Geometry: final body of the model. Coordinates: model frame, mm. A direction names the side the tool comes from. Coordinates: 2 decimals unless noted, no trailing zeros. Write each loop counter-clockwise with the first axis right and the second up, starting at its lowest first coordinate (ties: lowest second). Pieces come first, ordered by that corner, then holes. Notation, with made-up numbers: (2, 13.5) -> (6, 13.5) arc R8 cw to (6, 17.5) -> close; hole circle Ø9 at (-12, 62.5). An arc over 180 degrees is marked (long way). One line per item, written item: value.
```python
from build123d import *

# Parameters (mm, degrees)
SKETCH1_W            = 133
SKETCH1_H            = 41
BOSS_EXTRUDE1_DEPTH  = 12
SKETCH2_W            = 95
SKETCH2_H            = 12
BOSS_EXTRUDE2_DEPTH  = 15
FILLET1_R            = 2
M2_CLEARANCE_HOLE1_D = 2.4
VENT1_DEPTH          = 12
FILLET2_R            = 1


# Read off the part's stored shape, not the designer's step: Vent1
with BuildPart() as part:
    # Sketch1 → Boss-Extrude1 (new body)
    with BuildSketch(Plane.XY):
        Rectangle(SKETCH1_W, SKETCH1_H)
    extrude(amount=BOSS_EXTRUDE1_DEPTH)

    # Sketch2 → Boss-Extrude2 (add)
    with BuildSketch(Plane(origin=(0, 20.5, 0), x_dir=(1, 0, 0), z_dir=(0, 1, 0))):
        with Locations((-2, -6)):
            Rectangle(SKETCH2_W, SKETCH2_H)
    extrude(amount=BOSS_EXTRUDE2_DEPTH)

    # Fillet1
    fillet1_edges = [part.edges().sort_by_distance(p)[0] for p in [
        (-49.5, 35.5, 6),
        (45.5, 35.5, 6),
        (-66.5, 20.5, 6),
        (66.5, 20.5, 6),
        (66.5, -20.5, 6),
        (-66.5, -20.5, 6),
    ]]
    fillet(fillet1_edges, radius=FILLET1_R)

    # M2 Clearance Hole1 (through all)
    with Locations(Plane(origin=(-42, 27, 12), x_dir=(1, 0, 0), z_dir=(0, 0, 1))):
        with Locations((0, 0), (80, 0)):
            Hole(M2_CLEARANCE_HOLE1_D / 2)

    # Vent1 outline → Vent1 (cut)
    with BuildSketch(Plane.XY):
        Polygon((-39.847390778, 12.5), (-46.320873948, 12.5), (-58.5, 0.320873948), (-58.5, -6.152609222), align=None)
        Polygon((-26.302839797, 12.5), (-32.776322967, 12.5), (-57.776322967, -12.5), (-51.302839797, -12.5), align=None)
        Polygon((-12.758288815, 12.5), (-19.231771985, 12.5), (-44.231771985, -12.5), (-37.758288815, -12.5), align=None)
        Polygon((0.786262167, 12.5), (-5.687221003, 12.5), (-30.687221003, -12.5), (-24.213737833, -12.5), align=None)
        Polygon((14.330813149, 12.5), (7.857329979, 12.5), (-17.142670021, -12.5), (-10.669186851, -12.5), align=None)
        Polygon((27.875364131, 12.5), (21.401880961, 12.5), (-3.598119039, -12.5), (2.875364131, -12.5), align=None)
        Polygon((-53.39194176, 12.5), (-58.5, 12.5), (-58.5, 7.39194176), align=None)
        Polygon((41.419915112, 12.5), (34.946431942, 12.5), (9.946431942, -12.5), (16.419915112, -12.5), align=None)
        Polygon((54.964466094, 12.5), (48.490982924, 12.5), (23.490982924, -12.5), (29.964466094, -12.5), align=None)
        Polygon((37.035533906, -12.5), (43.509017076, -12.5), (58.5, 2.490982924), (58.5, 8.964466094), align=None)
        Polygon((50.580084888, -12.5), (58.5, -12.5), (58.5, -4.580084888), align=None)
    extrude(amount=VENT1_DEPTH, mode=Mode.SUBTRACT)

    # Fillet2
    fillet2_edges = [part.edges().sort_by_distance(p)[0] for p in [
        (50.580084888, -12.5, 6),
        (43.509017076, -12.5, 6),
        (58.5, 2.490982924, 6),
        (58.5, -4.580084888, 6),
        (37.035533906, -12.5, 6),
        (29.964466094, -12.5, 6),
        (54.964466094, 12.5, 6),
        (58.5, 8.964466094, 6),
        (23.490982924, -12.5, 6),
        (16.419915112, -12.5, 6),
        (41.419915112, 12.5, 6),
        (48.490982924, 12.5, 6),
        (9.946431942, -12.5, 6),
        (2.875364131, -12.5, 6),
        (27.875364131, 12.5, 6),
        (34.946431942, 12.5, 6),
        (14.330813149, 12.5, 6),
        (21.401880961, 12.5, 6),
        (-3.598119039, -12.5, 6),
        (-10.669186851, -12.5, 6),
        (0.786262167, 12.5, 6),
        (7.857329979, 12.5, 6),
        (-17.142670021, -12.5, 6),
        (-24.213737833, -12.5, 6),
        (-12.758288815, 12.5, 6),
        (-5.687221003, 12.5, 6),
        (-30.687221003, -12.5, 6),
        (-37.758288815, -12.5, 6),
        (-26.302839797, 12.5, 6),
        (-19.231771985, 12.5, 6),
        (-44.231771985, -12.5, 6),
        (-51.302839797, -12.5, 6),
        (-39.847390778, 12.5, 6),
        (-32.776322967, 12.5, 6),
        (-57.776322967, -12.5, 6),
        (-58.5, -6.152609222, 6),
        (-53.39194176, 12.5, 6),
        (-46.320873948, 12.5, 6),
        (-58.5, 0.320873948, 6),
        (-58.5, 7.39194176, 6),
        (58.5, -12.5, 6),
    ]]
    fillet(fillet2_edges, radius=FILLET2_R)


solid = part.part
```
(1) Pull-direction query (X, two-part tool) for faces 1 (the flat face through (-49.5, 27, 6)), 2 (the flat face through (51, 12.5, 6)), 3 (the flat face through (9.8, 0.9, 5.9)), 4 (the flat face through (-1, 8, 12)); classes: released by +X, released by -X, zero draft, split by the parting line, or undercut.
Responses:
face 1: released by -X
face 2: undercut
face 3: undercut
face 4: zero draft
(2) Section B-B (z = 1.5). State how many separate pieces and enclosed holes the cut face has, then the cut area to 3 significant figures.
Responses:
separate pieces: 1
enclosed holes: 13
area: 5,500 mm2
(3) Reachability of faces 5 (the flat face through (-44.408, 0.868, 5.916)), 6 (the flat face through (55, 20.5, 6)), 7 (the flat face through (-66.5, 0, 6)) from +Z, -Z, +X, -X, +Y, -Y: full face, straight path, thin tool, end or side. Return the list, or none.
Responses:
face 5: +Z, -Z
face 6: +Z, -Z, +X, +Y
face 7: +Z, -Z, -X, +Y, -Y
(4) Section A-A (y = 27). Return the cut outline in (x, z).
Responses:
outline: (-49.5, 0) -> (-43.2, 0) -> (-43.2, 12) -> (-49.5, 12) -> close; (-40.8, 0) -> (36.8, 0) -> (36.8, 12) -> (-40.8, 12) -> close; (39.2, 0) -> (45.5, 0) -> (45.5, 12) -> (39.2, 12) -> close
(5) Line query: line 1 (Y direction, x = -22, z = 4.5); line 2 (Y direction, x = 31, z = 7); line 3 (Y direction, x = -42, z = 9.5). Output: solid intervals per line, ascending. Write a range as [from, to].
Responses:
line 1: y = [-20.5, -10.29], [-3.81, 3.26], [9.73, 35.5]
line 2: y = [-20.5, -11.46], [-4.99, 2.08], [8.55, 35.5]
line 3: y = [-20.5, -12.48], [-10.27, -3.2], [3.28, 10.35], [12.47, 25.8], [28.2, 35.5]
(6) First-contact query: pin 1 (3 mm diameter, centred on x = -53.5, z = 3.5, fed in from +Y). Flat tip, straight axial feed; report the tip coordinate or a pass-through.
Responses:
pin 1: stops at y = 20.5
